Can you work these out from the drawing? Everything is in mm from the part's minimum corner. Round coordinates to 2 decimals unless told otherwise and drop trailing zeros. Write each loop counter-clockwise with the first axis right and the second up, starting at its lowest first coordinate (ties: lowest second). Pieces come first, ordered by that corner, then holes. Notation, with made-up numbers: (53.5, 73.5) - (81.5, 73.5) arc R28 ccw to (81.5, 110.5) - close; hole circle Ø4 at (45.25, 30.25). An arc over 180 degrees is marked (long way). Write each question's results on one line, items separated by ' | '. Start each with the question number.
(1) Imagine slicing it at B-B on x = 5.5. Write out the boundary of the cut face in (y, z), then the cut area to 3 significant figures.
(2) Imagine slicing it at C-C on z = 11. Write out the boundary of the cut face in (x, y).
(3) Please list where these lines run through material, in increasing order: line 1 (Z direction, x = 5.5, y = 0.8); line 2 (X direction, y = 2.45, z = 25); line 3 (Z direction, x = 13.5, y = 0.75). Write a range as [from, to].
(4) Imagine slicing it at D-D on y = 1.65. Write out the boundary of the cut face in (x, z).
(5) Imagine slicing it at A-A on z = 18. Write out the boundary of the cut face in (x, y), then the cut area to 3 significant figures.
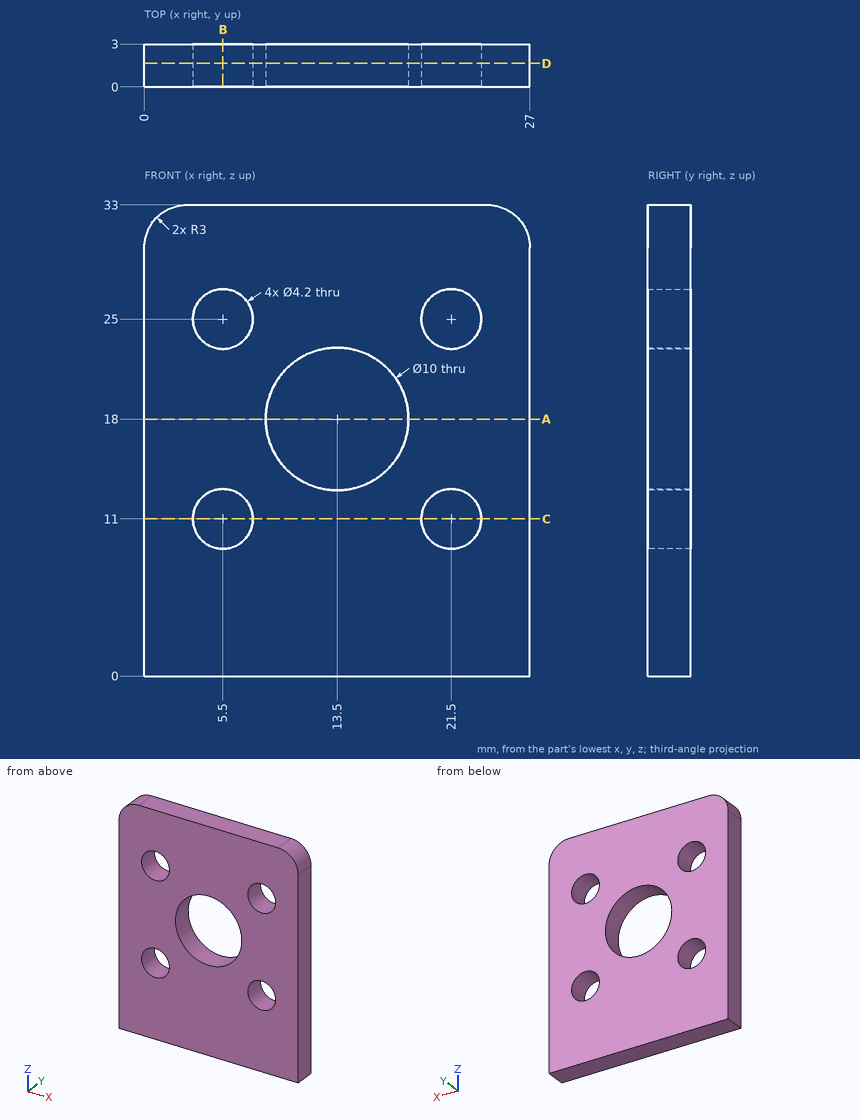
Response:
1) outline: (0, 0) - (3, 0) - (3, 8.9) - (0, 8.9) - close; (0, 13.1) - (3, 13.1) - (3, 22.9) - (0, 22.9) - close; (0, 27.1) - (3, 27.1) - (3, 33) - (0, 33) - close | area: 73.8 mm²
2) outline: (0, 0) - (3.4, 0) - (3.4, 3) - (0, 3) - close; (7.6, 0) - (19.4, 0) - (19.4, 3) - (7.6, 3) - close; (23.6, 0) - (27, 0) - (27, 3) - (23.6, 3) - close
3) line 1: [0, 8.9], [13.1, 22.9], [27.1, 33] | line 2: [0, 3.4], [7.6, 19.4], [23.6, 27] | line 3: [0, 13], [23, 33]
4) outline: (0, 0) - (27, 0) - (27, 30) arc R3 ccw to (24, 33) - (3, 33) arc R3 ccw to (0, 30) - close; hole circle Ø4.2 at (5.5, 11); hole circle Ø4.2 at (5.5, 25); hole circle Ø10 at (13.5, 18); hole circle Ø4.2 at (21.5, 11); hole circle Ø4.2 at (21.5, 25)
5) outline: (0, 0) - (8.5, 0) - (8.5, 3) - (0, 3) - close; (18.5, 0) - (27, 0) - (27, 3) - (18.5, 3) - close | area: 51.0 mm²
